from build123d import *

# Parameters (mm, degrees)
F0_R     = 0.975
F0_W     = 36.6
F0_H     = 0.7
F0_W_2   = 0.7
F0_H_2   = 36.6
F0_H_3   = 12.8
F0_H_4   = 12.3
F0_H_5   = 11.5
F1_DEPTH = 1.2
F2_DEPTH = 1.75
F3_DEPTH = 4
F4_R     = 1.8
F5_SIZE  = 0.5


with BuildPart() as f1:
    # F0 (on Top) → F1 (new body)
    with BuildSketch(Plane.XY):
        Polygon((18.3, 6), (18.3, 18.3), (-18.3, 18.3), (-18.3, -18.3), (18.3, -18.3), (18.3, -5.5), align=None)
        with Locations((-16.625, -16.625)):
            Circle(F0_R, mode=Mode.SUBTRACT)
        with Locations((11.775, -5.975)):
            Circle(F0_R, mode=Mode.SUBTRACT)
        with Locations((-16.625, 16.625)):
            Circle(F0_R, mode=Mode.SUBTRACT)
        with Locations((0, 18.65)):
            Rectangle(F0_W, F0_H)
        with Locations((0, -18.65)):
            Rectangle(F0_W, F0_H)
        with Locations((-18.65, 0)):
            Rectangle(F0_W_2, F0_H_2)
        with Locations((18.65, -11.9)):
            Rectangle(F0_W_2, F0_H_3)
        with Locations((18.65, 12.15)):
            Rectangle(F0_W_2, F0_H_4)
        with Locations((18.65, 0.25)):
            Rectangle(F0_W_2, F0_H_5)
        with Locations((11.775, -5.975)):
            Circle(F0_R)
        with Locations((-16.625, -16.625)):
            Circle(F0_R)
        with Locations((-16.625, 16.625)):
            Circle(F0_R)
        with Locations((18.65, 18.65)):
            Rectangle(F0_W_2, F0_H)
        with Locations((-18.65, 18.65)):
            Rectangle(F0_W_2, F0_H)
        with Locations((18.65, -18.65)):
            Rectangle(F0_W_2, F0_H)
        with Locations((-18.65, -18.65)):
            Rectangle(F0_W_2, F0_H)
    extrude(amount=-F1_DEPTH)

    # F0 (on Top) → F2 (join)
    with BuildSketch(Plane.XY):
        with Locations((0, 18.65)):
            Rectangle(F0_W, F0_H)
        with Locations((-18.65, 18.65)):
            Rectangle(F0_W_2, F0_H)
        with Locations((18.65, 18.65)):
            Rectangle(F0_W_2, F0_H)
        with Locations((18.65, 12.15)):
            Rectangle(F0_W_2, F0_H_4)
        with Locations((18.65, -11.9)):
            Rectangle(F0_W_2, F0_H_3)
        with Locations((18.65, -18.65)):
            Rectangle(F0_W_2, F0_H)
        with Locations((0, -18.65)):
            Rectangle(F0_W, F0_H)
        with Locations((-18.65, -18.65)):
            Rectangle(F0_W_2, F0_H)
        with Locations((-18.65, 0)):
            Rectangle(F0_W_2, F0_H_2)
    extrude(amount=F2_DEPTH)

    # F0 (on Top) → F3 (join)
    with BuildSketch(Plane.XY):
        with Locations((-16.625, 16.625)):
            Circle(F0_R)
        with Locations((-16.625, -16.625)):
            Circle(F0_R)
        with Locations((11.775, -5.975)):
            Circle(F0_R)
    extrude(amount=F3_DEPTH)

    # F4
    f4_edges = [f1.edges().sort_by_distance(p)[0] for p in [
        (-19, 19, 0.275),
        (19, 19, 0.275),
        (-19, -19, 0.275),
        (19, -19, 0.275),
    ]]
    fillet(f4_edges, radius=F4_R)

    # F5
    f5_edges = [f1.edges().sort_by_distance(p)[0] for p in [
        (0, -19, -1.2),
        (10.8, -5.975, 4),
        (-17.6, 16.625, 4),
        (-17.6, -16.625, 4),
        (-17.6, 16.625, 0),
        (10.8, -5.975, 0),
        (-17.6, -16.625, 0),
    ]]
    chamfer(f5_edges, length=F5_SIZE)


solid = f1.part
Could you check a few things on this model? Use its own coordinates, in mm. A direction names the side the tool comes from. Give positions to 0.01 mm unless a question says otherwise; leave off trailing zeros. Write each loop counter-clockwise with the first axis right and the second up, starting at its lowest first coordinate (ties: lowest second). Pieces come first, ordered by that corner, then holes. Notation, with made-up numbers: (38.25, 41.25) - (74.25, 41.25) arc R22 ccw to (74.25, 49.25) - close; hole circle Ø11 at (2.25, 20). An arc over 180 degrees is marked (long way). Use CSV: the item, a comma, the result in double quotes. Start each with the question number.
Item 1: I want a section at A-A, the plane y = 3. Please give me the cut outline in (x, z), then the cut area to 3 significant figures.
Item 2: For faces 1 (the face through (0, 0, 0)), 2 (the face through (-16.6, -16.6, 4)), which set-ups out of +Z, -Z, +X, -X, +Y, -Y let a thin tool reach every point of the face, with its end or its side?
Item 3: I'm going to push flat-ended pins straight in: pin 1 (0.6 mm diameter, centred on x = 18.5, z = 1, fed in from +Y); pin 2 (1 mm diameter, centred on x = 0, y = 10.5, fed in from +Z); pin 3 (1 mm diameter, centred on x = 10, z = 2.5, fed in from +Y); pin 4 (0.8 mm diameter, centred on x = 18.5, z = 1, fed in from -Y). Where does each tip first touch, or does it pass through?
Item 4: If I drill on line 1 along Y through (x, z) = (-4, 0.65); line 2 along Z through (x, y) = (-2.5, -11); line 3 along X through (y, z) = (2, 1.25), over which ranges is the centre line in solid material (lowest first)?
Item 5: If we mould it in two halves opening along Y, with no side actions, what happens to faces 3 (the face through (-18.487, -18.459, 0.542)), 4 (the face through (0, 0, -1.2)), 5 (the face through (-15.695, 16.918, 1.979))? For each: pulls with the +Y half, pulls with the -Y half, needs draft (parallel to the pull), parting line crosses it, or undercut.
Item 6: I want a section at B-B, the plane x = -6.5. Please give me the cut outline in (y, z).
Item 7: I want a section at C-C, the plane z = 2.4. Please give me the cut outline in (x, y) (3 decimals), then the cut area to 3 significant figures.
Findings:
1,outline,"(-19, -0.7) - (-18.5, -1.2) - (18.5, -1.2) - (19, -0.7) - (19, 0) - (-18.3, 0) - (-18.3, 1.75) - (-19, 1.75) - close"
1,area,"46.6 mm2"
2,face 1,"+Z"
2,face 2,"+Z, +X, -X, +Y, -Y"
3,pin 1,"stops at y = 18.7"
3,pin 2,"stops at z = 0"
3,pin 3,"passes through"
3,pin 4,"stops at y = -18.76"
4,line 1,"y = -19 to -18.3, 18.3 to 19"
4,line 2,"z = -1.2 to 0"
4,line 3,"x = -19 to -18.3"
5,face 3,"pulls with the -Y half"
5,face 4,"needs draft"
5,face 5,"undercut"
6,outline,"(-19, -0.7) - (-18.5, -1.2) - (18.5, -1.2) - (19, -0.7) - (19, 1.75) - (18.3, 1.75) - (18.3, 0) - (-18.3, 0) - (-18.3, 1.75) - (-19, 1.75) - close"
7,outline,"circle Ø1.95 at (-16.625, -16.625); circle Ø1.95 at (-16.625, 16.625); circle Ø1.95 at (11.775, -5.975)"
7,area,"8.96 mm2"
